```python
from build123d import *

# Parameters (mm, degrees)
SKETCH1_R                       = 1.5875
BOSS_EXTRUDE1_DEPTH             = 3.175
SKETCH2_R                       = 13.97
CUT_EXTRUDE1_DEPTH              = 1.778
F_9_64_0_14063_DIAMETER_HOLE1_D = 3.572002


with BuildPart() as part:
    # Sketch1 → Boss-Extrude1 (new body)
    with BuildSketch(Plane(origin=(0, 0, 0), x_dir=(1, 0, 0), z_dir=(0, 1, 0))):
        with BuildLine():
            Line((139.17898319, 28.575), (152.4, 28.575))
            Line((152.4, 28.575), (152.4, 0))
            Line((152.4, 0), (0, 0))
            Line((0, 0), (0, 28.575))
            Line((0, 28.575), (13.72901681, 28.575))
            add(Edge.make_bspline(
                [(13.72901681, 28.575), (17.042474439, 27.940707838), (17.145, 26.4414)],
                knots=[0, 0, 0, 0.606076244, 0.606076244, 0.606076244], degree=2))
            ThreePointArc((17.145, 26.4414), (19.05, 24.5364), (20.955, 26.4414))
            add(Edge.make_bspline(
                [(24.37098319, 28.575), (21.057525561, 27.940707838), (20.955, 26.4414)],
                knots=[0, 0, 0, 0.606076244, 0.606076244, 0.606076244], degree=2))
            Line((24.37098319, 28.575), (42.43101681, 28.575))
            add(Edge.make_bspline(
                [(42.43101681, 28.575), (45.744474439, 27.940707838), (45.847, 26.4414)],
                knots=[0, 0, 0, 0.606076244, 0.606076244, 0.606076244], degree=2))
            ThreePointArc((45.847, 26.4414), (47.752, 24.5364), (49.657, 26.4414))
            add(Edge.make_bspline(
                [(53.07298319, 28.575), (49.759525561, 27.940707838), (49.657, 26.4414)],
                knots=[0, 0, 0, 0.606076244, 0.606076244, 0.606076244], degree=2))
            Line((53.07298319, 28.575), (71.13301681, 28.575))
            add(Edge.make_bspline(
                [(71.13301681, 28.575), (74.446474439, 27.940707838), (74.549, 26.4414)],
                knots=[0, 0, 0, 0.606076244, 0.606076244, 0.606076244], degree=2))
            ThreePointArc((74.549, 26.4414), (76.454, 24.5364), (78.359, 26.4414))
            add(Edge.make_bspline(
                [(81.77498319, 28.575), (78.461525561, 27.940707838), (78.359, 26.4414)],
                knots=[0, 0, 0, 0.606076244, 0.606076244, 0.606076244], degree=2))
            Line((81.77498319, 28.575), (99.83501681, 28.575))
            add(Edge.make_bspline(
                [(99.83501681, 28.575), (103.148474439, 27.940707838), (103.251, 26.4414)],
                knots=[0, 0, 0, 0.606076244, 0.606076244, 0.606076244], degree=2))
            ThreePointArc((103.251, 26.4414), (105.156, 24.5364), (107.061, 26.4414))
            add(Edge.make_bspline(
                [(110.47698319, 28.575), (107.163525561, 27.940707838), (107.061, 26.4414)],
                knots=[0, 0, 0, 0.606076244, 0.606076244, 0.606076244], degree=2))
            Line((110.47698319, 28.575), (128.53701681, 28.575))
            add(Edge.make_bspline(
                [(128.53701681, 28.575), (131.850474439, 27.940707838), (131.953, 26.4414)],
                knots=[0, 0, 0, 0.606076244, 0.606076244, 0.606076244], degree=2))
            ThreePointArc((131.953, 26.4414), (133.858, 24.5364), (135.763, 26.4414))
            add(Edge.make_bspline(
                [(139.17898319, 28.575), (135.865525561, 27.940707838), (135.763, 26.4414)],
                knots=[0, 0, 0, 0.606076244, 0.606076244, 0.606076244], degree=2))
        make_face()
        with Locations(Location((19.05, 17.0434, 0), (0, 0, 270))):
            Circle(SKETCH1_R, mode=Mode.SUBTRACT)
        with Locations(Location((47.625, 17.0434, 0), (0, 0, 270))):
            Circle(SKETCH1_R, mode=Mode.SUBTRACT)
        with Locations(Location((76.2, 17.0434, 0), (0, 0, 270))):
            Circle(SKETCH1_R, mode=Mode.SUBTRACT)
        with Locations(Location((104.775, 17.0434, 0), (0, 0, 270))):
            Circle(SKETCH1_R, mode=Mode.SUBTRACT)
        with Locations(Location((133.35, 17.0434, 0), (0, 0, 270))):
            Circle(SKETCH1_R, mode=Mode.SUBTRACT)
    extrude(amount=BOSS_EXTRUDE1_DEPTH)

    # Sketch2 → Cut-Extrude1 (cut)
    with BuildSketch(Plane.XZ):
        with Locations((19.05, -17.0434)):
            Circle(SKETCH2_R)
        with Locations((47.625, -17.0434)):
            Circle(SKETCH2_R)
        with Locations((76.2, -17.0434)):
            Circle(SKETCH2_R)
        with Locations((104.775, -17.0434)):
            Circle(SKETCH2_R)
        with Locations((133.35, -17.0434)):
            Circle(SKETCH2_R)
    extrude(amount=-CUT_EXTRUDE1_DEPTH, mode=Mode.SUBTRACT)

    # 9/64 (0.14063) Diameter Hole1 (through all)
    with Locations(Plane(origin=(0, 3.175, 0), x_dir=(1, 0, 0), z_dir=(0, 1, 0))):
        with Locations((3.175, 25.4), (3.175, 3.175), (149.225, 3.175), (149.225, 25.4)):
            Hole(F_9_64_0_14063_DIAMETER_HOLE1_D / 2)


solid = part.part
```
Work out the finished part from the listing and answer in its coordinate system (mm). A direction names the side the tool comes from. Round coordinates to 2 decimals unless told otherwise and drop trailing zeros. Write each loop counter-clockwise with the first axis right and the second up, starting at its lowest first coordinate (ties: lowest second). Pieces come first, ordered by that corner, then holes.
1) Which of the six approach directions +Z, -Z, +X, -X, +Y, -Y give full straight-line access (tool end or side, diameter ignored) to faces 1 (the face through (91, 2, -28.575)), 2 (the face through (76.697, 0.877, -3.082))?
2) A cutting plane is placed at B-B on y = 1.1. Determine the outline of the cut face in (x, z) (3 decimals).
3) Determine the mould class of faces 3 (the face through (3.562, 1.565, -23.656)), 4 (the face through (0, 2, -14)), 5 (the face through (7, 2, -28.575)) for opening direction Z: pulls with the +Z half, pulls with the -Z half, needs draft (parallel to the pull), parting line crosses it, or undercut.
4) A cutting plane is placed at C-C on x = 133.35. Determine the outline of the cut face in (y, z) (3 decimals).
5) Consider probe 1 along X at (y, z) = (0.6, -5); probe 2 along X at (y, z) = (2, -24); probe 3 along X at (y, z) = (2.5, -18). Determine where each line is inside the solid, lowest interval first.
6) A cutting plane is placed at A-A on x = 19.05. Determine the outline of the cut face in (y, z) (3 decimals).
7) Flat-ended cylindrical pins translate along their axes: P1, Ø3, axis at x = 43, z = -12, coming from the -Y side; P2, Ø1.5, axis at x = 75, y = 2, coming from the -Z side. Find the tip coordinate at first contact, or state that the pin passes through.
Entries:
1. face 1: -Z, +X, -X, +Y, -Y
1. face 2: -Y
2. outline: (0, -28.575) - (11.164, -28.575) arc R13.97 cw (long way) to (26.936, -28.575) - (39.739, -28.575) arc R13.97 cw (long way) to (55.511, -28.575) - (68.314, -28.575) arc R13.97 cw (long way) to (84.086, -28.575) - (96.889, -28.575) arc R13.97 cw (long way) to (112.661, -28.575) - (125.464, -28.575) arc R13.97 cw (long way) to (141.236, -28.575) - (152.4, -28.575) - (152.4, 0) - (0, 0) - close; hole circle Ø3.572 at (3.175, -25.4); hole circle Ø3.572 at (3.175, -3.175); hole circle Ø3.572 at (149.225, -25.4); hole circle Ø3.572 at (149.225, -3.175)
3. face 3: undercut
3. face 4: needs draft
3. face 5: pulls with the -Z half
4. outline: (0, -3.073) - (1.778, -3.073) - (1.778, -15.456) - (3.175, -15.456) - (3.175, 0) - (0, 0) - close; (1.778, -24.605) - (3.175, -24.605) - (3.175, -18.631) - (1.778, -18.631) - close
5. probe 1: x = 0 to 11.97, 26.13 to 40.55, 54.7 to 69.12, 83.28 to 97.7, 111.85 to 126.27, 140.43 to 152.4
5. probe 2: x = 0 to 2.07, 4.28 to 148.12, 150.33 to 152.4
5. probe 3: x = 0 to 17.78, 20.32 to 46.36, 48.89 to 74.93, 77.47 to 103.51, 106.04 to 132.08, 134.62 to 152.4
6. outline: (0, -3.073) - (1.778, -3.073) - (1.778, -15.456) - (3.175, -15.456) - (3.175, 0) - (0, 0) - close; (1.778, -24.536) - (3.175, -24.536) - (3.175, -18.631) - (1.778, -18.631) - close
7. P1: stops at y = 1.78
7. P2: stops at z = -27.2
